Here's how the part is built. I have some questions about the finished solid (model axes, mm). A direction names the side the tool comes from. Round coordinates to 2 decimals unless told otherwise and drop trailing zeros. Write each loop counter-clockwise with the first axis right and the second up, starting at its lowest first coordinate (ties: lowest second). Pieces come first, ordered by that corner, then holes. Notation, with made-up numbers: (51, 28) - (90, 28) arc R17 cw to (90, 40) - close; hole circle Ø9 at (-21.75, -36.75). An arc over 180 degrees is marked (long way). Write item = value, one per line. Start each with the question number.
Item 1: For P1, Ø1, axis at y = -4, z = -1, coming from the -X side (3 decimals); P2, Ø1, axis at y = 4.5, z = -1, coming from the +X side (3 decimals), each with a flat end and sliding along its axis, tell me the tip position at first contact or that it passes through.
Item 2: If we section it at A-A (y = -3.25): Please give me the cut outline in (x, z) (3 decimals).
Item 3: If we section it at D-D (z = -1): Give the number of separate pieces and of enclosed holes in the cut face, and give its area (3 significant figures).
Item 4: Which directions (+Z, -Z, +X, -X, +Y, -Y) give clear straight access to the entire face, cutting with the end or side of a thin tool? Please do faces 1 (the face through (0, 3.555, 0)), 2 (the face through (0, 0, -0.705)), 3 (the face through (0.335, -4.034, -0.754)), 4 (the face through (2.205, 4.034, -0.754)), 5 (the face through (-0.335, 4.034, -0.754)).
Item 5: If I drill on line 1 along Z through (x, y) = (-2, 2.25) (3 decimals); line 2 along Y through (x, z) = (2, 0.25) (3 decimals); line 3 along Z through (x, y) = (-3.25, -1) (3 decimals), over which ranges is the centre line in solid material (lowest first)? Write a range as [from, to].
Item 6: If we section it at C-C (z = 0.35): Please give me the cut outline in (x, y) (3 decimals).
```python
from build123d import *

# Parameters (mm, degrees)
F0_W     = 7.62
F0_H     = 7.11
F1_DEPTH = 0.705
F3_DEPTH = 0.66
F5_DEPTH = 25
F6_R     = 0.01
F7_R     = 0.3408088795
F8_DEPTH = 0.1
F9_R     = 0.09999
F11_W    = 0.6
F11_H    = 0.35
F13_R    = 0.1
F14_W    = 0.6
F14_H    = 0.3504652178
F16_R    = 0.15


# Not quite as in the source:
# - a fillet or chamfer is up to 0.001 mm smaller than in the source, because OpenCascade refuses the exact size
# - a feature names something its author has since deleted; it is built from what else it names


with BuildPart() as f1:
    # F0 (on Top) → F1 (new body, symmetric)
    with BuildSketch(Plane.XY):
        Rectangle(F0_W, F0_H)
    extrude(amount=F1_DEPTH, both=True)

    # F2 (on face) → F3 (join)
    with BuildSketch(Plane(origin=(0, 0, -0.705), x_dir=(1, 0, 0), z_dir=(0, 0, -1))):
        Polygon((-3.81, 2.81), (-3.81, 0), (-3.81, -2.81), (-3.15, -2.81), (-3.15, 2.81), align=None)
        Polygon((3.81, 0), (3.81, 2.81), (3.15, 2.81), (3.15, -2.81), (3.81, -2.81), align=None)
    extrude(amount=F3_DEPTH)

    # F4 (on face) → F5 (cut)
    with BuildSketch(Plane(origin=(-3.81, 0, 0), x_dir=(0, -1, 0), z_dir=(-1, 0, 0))):
        Polygon((-2.81, -1.365), (-2.6863825042, -1.365), (-2.81, -0.705), align=None)
        Polygon((2.81, -1.365), (2.81, -0.705), (2.6863825042, -1.365), align=None)
    extrude(amount=-F5_DEPTH, mode=Mode.SUBTRACT)

    # F6
    f6_edges = [f1.edges().sort_by_distance(p)[0] for p in [
        (-3.81, 0, 0.705),
        (-3.81, -3.555, 0),
        (0, -3.555, 0.705),
        (-3.81, 3.555, 0),
        (3.81, -3.555, 0),
        (3.81, 0, 0.705),
        (3.81, 3.555, 0),
        (0, 3.555, 0.705),
        (0, 3.555, -0.705),
        (0, -3.555, -0.705),
        (3.81, -3.1825, -0.705),
        (3.81, -2.748191, -1.035),
        (3.81, 2.748191, -1.035),
        (3.81, 3.1825, -0.705),
        (-3.81, -2.748191, -1.035),
        (-3.81, -3.1825, -0.705),
        (-3.81, 3.1825, -0.705),
        (-3.81, 2.748191, -1.035),
    ]]
    fillet(f6_edges, radius=F6_R)

    # F7 (on face) → F8 (cut)
    with BuildSketch(Plane.XY.offset(0.705)):
        with Locations((-2.9591911205, -2.7141911205)):
            Circle(F7_R)
    extrude(amount=-F8_DEPTH, mode=Mode.SUBTRACT)

    # F9 (radius 0.1 in the source; OpenCascade refuses exactly that, so slightly less here)
    f9_edges = [f1.edges().sort_by_distance(p)[0] for p in [
        (-3.3, -2.714191, 0.605),
    ]]
    fillet(f9_edges, radius=F9_R)

    # F12: sweep along a path in F10
    with BuildLine(Plane.YZ) as f12_path:
        Line((3.555, 0), (3.955, 0))
        Line((3.955, 0), (4.165, -1.5318583786))
        Line((4.165, -1.5318583786), (4.765, -1.535))
    # F11 (on face) → F12 (sweep)
    with BuildSketch(Plane(origin=(0, 3.555, 0), x_dir=(-1, 0, 0), z_dir=(0, 1, 0))):
        with Locations((-1.905, 0)):
            Rectangle(F11_W, F11_H)
        with Locations((-0.635, 0)):
            Rectangle(F11_W, F11_H)
        with Locations((0.635, 0)):
            Rectangle(F11_W, F11_H)
        with Locations((1.905, 0)):
            Rectangle(F11_W, F11_H)
    sweep(path=f12_path.line, transition=Transition.RIGHT)

    # F13
    f13_edges = [f1.edges().sort_by_distance(p)[0] for p in [
        (-1.905, 4.107646, 0.175),
        (-1.905, 4.317756, -1.357656),
        (-0.635, 4.107646, 0.175),
        (-0.635, 4.317756, -1.357656),
        (0.635, 4.107646, 0.175),
        (0.635, 4.317756, -1.357656),
        (1.905, 4.107646, 0.175),
        (1.905, 4.317756, -1.357656),
        (1.905, 3.802354, -0.175),
        (0.635, 3.802354, -0.175),
        (-0.635, 3.802354, -0.175),
        (-1.905, 3.802354, -0.175),
        (-1.905, 4.012244, -1.706061),
        (-0.635, 4.012244, -1.706061),
        (0.635, 4.012244, -1.706061),
        (1.905, 4.012244, -1.706061),
    ]]
    fillet(f13_edges, radius=F13_R)

    # F15: sweep along a path in F10
    with BuildLine(Plane.YZ) as f15_path:
        Line((-3.555, 0), (-3.955, 0))
        Line((-3.955, 0), (-4.165, -1.5318583786))
        Line((-4.165, -1.5318583786), (-4.765, -1.535))
    # F14 (on face) → F15 (sweep)
    with BuildSketch(Plane.XZ.offset(3.555)):
        with Locations((-1.905, 0)):
            Rectangle(F14_W, F14_H)
        with Locations((-0.635, 0)):
            Rectangle(F14_W, F14_H)
        with Locations((0.635, 0)):
            Rectangle(F14_W, F14_H)
        with Locations((1.905, 0)):
            Rectangle(F14_W, F14_H)
    sweep(path=f15_path.line, transition=Transition.RIGHT)

    # F16
    f16_edges = [f1.edges().sort_by_distance(p)[0] for p in [
        (-1.905, -4.107849, 0.175233),
        (-0.635, -4.107849, 0.175233),
        (0.635, -4.107849, 0.175233),
        (1.905, -4.107849, 0.175233),
        (-1.905, -4.317959, -1.357424),
        (-0.635, -4.317959, -1.357424),
        (0.635, -4.317959, -1.357424),
        (1.905, -4.317959, -1.357424),
        (-1.905, -3.802151, -0.175233),
        (-0.635, -3.802151, -0.175233),
        (0.635, -3.802151, -0.175233),
        (1.905, -3.802151, -0.175233),
        (0.635, -4.012041, -1.706292),
        (-0.635, -4.012041, -1.706292),
        (-1.905, -4.012041, -1.706292),
        (1.905, -4.012041, -1.706292),
    ]]
    fillet(f16_edges, radius=F16_R)


solid = f1.part
```
Reply:
q1.P1 = -2.205
q1.P2 = 2.205
q2.outline = (-3.81, -0.695) arc R0.01 ccw to (-3.8, -0.705) - (3.8, -0.705) arc R0.01 ccw to (3.81, -0.695) - (3.81, 0.695) arc R0.01 ccw to (3.8, 0.705) - (-3.8, 0.705) arc R0.01 ccw to (-3.81, 0.695) - close
q3.separate_pieces = 10
q3.enclosed_holes = 0
q3.area = 8.97 mm2
q4.face_1 = none
q4.face_2 = -Z
q4.face_3 = +Z, -Z, -Y
q4.face_4 = +Z, -Z, +X, +Y
q4.face_5 = +Z, -Z, +Y
q5.line_1 = [-0.705, 0.705]
q5.line_2 = [-3.555, 3.555]
q5.line_3 = [-1.365, 0.705]
q6.outline = (-3.81, -3.545) arc R0.01 ccw to (-3.8, -3.555) - (3.8, -3.555) arc R0.01 ccw to (3.81, -3.545) - (3.81, 3.545) arc R0.01 ccw to (3.8, 3.555) - (-3.8, 3.555) arc R0.01 ccw to (-3.81, 3.545) - close
